For this review, use the dimensioned drawing (mm, ordinates from the lowest corner) and the shaded views. A direction names the side the tool comes from. Round coordinates to 2 decimals unless told otherwise and drop trailing zeros. Order: outer loops, then holes, each group sorted by start corner. A loop starts at its lowest first (then second) coordinate and runs counter-clockwise, first axis right, second up. Notation, with made-up numbers: M 77.5,-7 L 106.5,-7 A4 ccw 106.5,0 Z; hole C -25.5,-36.75 d10. An arc over 180 degrees is marked long. Answer as CSV lines item,"result". Start each with the question number.
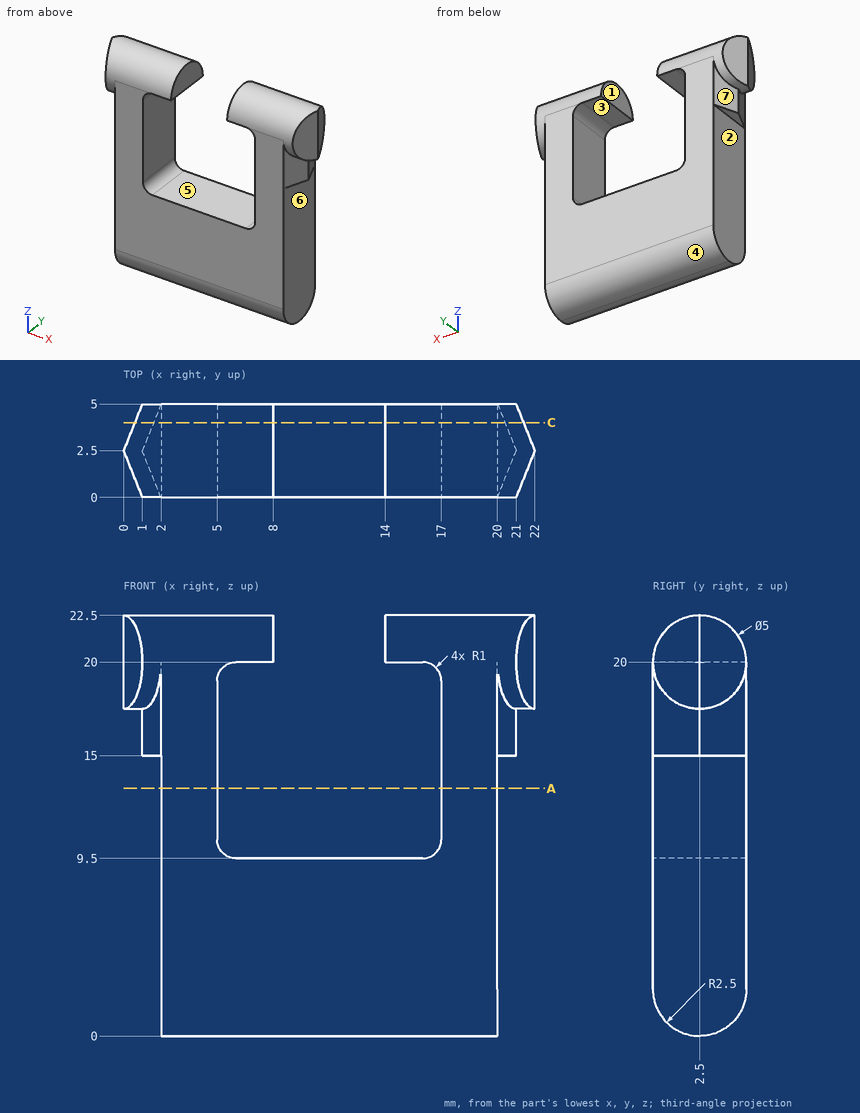
Item 1: Tool access review of the marked faces 5, 6 and 7: name each direction out of +Z, -Z, +X, -X, +Y, -Y from which nothing blocks a thin tool from reaching the whole face with its end or side.
Item 2: Wall thickness on probe 1 along Z at (x, y) = (6.25, 2.6); probe 2 along X at (y, z) = (1.15, 14); probe 3 along X at (y, z) = (4.15, 6): over which ranges is each line inside the solid? List them lowest first. Write a range as [from, to].
Item 3: Consider section A-A (z = 13.25). State the section outline as (x, y) points.
Item 4: The part is to be moulded in two halves that separate along X. For the marked faces 1, 2, 3 and 4, say which applies: +X half, -X half, draft (parallel to the pull), parting line (faces both ways), or undercut.
Item 5: Consider section C-C (y = 4). State the section outline as (x, z) points.
Item 6: For pin 1 (0.8 mm diameter, centred on x = 1.5, y = 3, fed in from -Z); pin 2 (2 mm diameter, centred on y = 0.5, z = 7, fed in from -X); pin 3 (3 mm diameter, centred on y = 2, z = 3.5, fed in from +X), all flat-tipped, find the tip position at first contact; note any pin that passes through.
Reported:
1,face 5,"+Y, -Y"
1,face 6,"-Z, +X, +Y, -Y"
1,face 7,"-Z, -X, +Y"
2,probe 1,"z = [0, 9.5], [20, 22.5]"
2,probe 2,"x = [2, 5], [17, 20]"
2,probe 3,"x = [2, 20]"
3,outline,"M 2,0 L 5,0 L 5,5 L 2,5 Z; M 17,0 L 20,0 L 20,5 L 17,5 Z"
4,face 1,"undercut"
4,face 2,"-X half"
4,face 3,"undercut"
4,face 4,"draft"
5,outline,"M 0.6,18 L 1.6,18 L 1.6,15 L 2,15 L 2,0.5 L 20,0.5 L 20,15 L 20.4,15 L 20.4,18 L 21.4,18 L 21.4,22 L 14,22 L 14,20 L 16,20 A1 cw 17,19 L 17,10.5 A1 cw 16,9.5 L 6,9.5 A1 cw 5,10.5 L 5,19 A1 cw 6,20 L 8,20 L 8,22 L 0.6,22 Z"
6,pin 1,"stops at z = 15"
6,pin 2,"stops at x = 2"
6,pin 3,"stops at x = 20"
